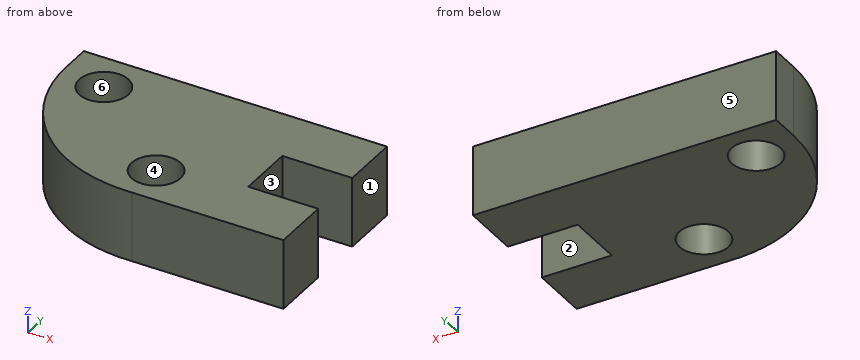
```python
from build123d import *

# Parameters (mm, degrees)
ESQUISSE1_R        = 2.1
BOSS_EXTRU_1_DEPTH = 6


with BuildPart() as part:
    # Esquisse1 → Boss.-Extru.1 (new body)
    with BuildSketch(Plane.XY):
        with BuildLine():
            Line((0, 0), (0, -5.05))
            Line((0, -5.05), (-6, -5.05))
            Line((-6, -5.05), (-6, -10))
            Line((-6, -10), (0, -10))
            Line((0, -10), (0, -15.05))
            Line((0, -15.05), (-13, -15.05))
            ThreePointArc((-13, -15.05), (-22.164162355, -11.534690089), (-26, -2.5))
            Line((-26, -2.5), (-26, 0))
            Line((-26, 0), (0, 0))
        make_face()
        with Locations((-22.2, -3.525)):
            Circle(ESQUISSE1_R, mode=Mode.SUBTRACT)
        with Locations((-13, -11.525)):
            Circle(ESQUISSE1_R, mode=Mode.SUBTRACT)
    extrude(amount=BOSS_EXTRU_1_DEPTH)


solid = part.part
```
Build history of the part. All positions in model axes, mm. Face numbers are marked on the shaded views. A direction names the side the tool comes from. Give positions to 0.01 mm unless a question says otherwise; leave off trailing zeros. Loops run counter-clockwise (first coordinate to the right, second up) from the corner with the lowest first, then second, coordinate; pieces in that order, holes last.
1) Band-saw the part on C-C on z = 2.7. List the corners of the cut face in (x, y) (3 decimals), then the cut area to 3 significant figures.
Values follow:
outline: (-26, -2.5) arc R12.558 ccw to (-13, -15.05) - (0, -15.05) - (0, -10) - (-6, -10) - (-6, -5.05) - (0, -5.05) - (0, 0) - (-26, 0) - close; hole circle Ø4.2 at (-22.2, -3.525); hole circle Ø4.2 at (-13, -11.525)
area: 300 mm2
2) Two-plate mould, pull along X, no slides. Class the marked faces 3, 4, 5 and 6: released by +X, released by -X, zero draft, split by the parting line, or undercut.
Values follow:
face 3: released by +X
face 4: undercut
face 5: zero draft
face 6: undercut
3) Band-saw the part on B-B on y = -12. List the corners of the cut face in (x, z).
Values follow:
outline: (-21.65, 0) - (-15.05, 0) - (-15.05, 6) - (-21.65, 6) - close; (-10.95, 0) - (0, 0) - (0, 6) - (-10.95, 6) - close
4) 3-axis set-ups, long thin cutter, end or side, ignore diameter. For the marked faces 1 and 2: which of +Z, -Z, +X, -X, +Y, -Y reach the whole face in a straight line?
Values follow:
face 1: +Z, -Z, +X, +Y, -Y
face 2: +Z, -Z, +X
5) Probe line 1 along Y through (x, z) = (-13, 4.9) (3 decimals); line 2 along Y through (x, z) = (-2.75, 2.25); line 3 along X through (y, z) = (-3.5, 5.2). List the from-to ranges inside material, lowest first.
Values follow:
line 1: y = -15.05 to -13.625, -9.425 to 0
line 2: y = -15.05 to -10, -5.05 to 0
line 3: x = -25.96 to -24.3, -20.1 to 0
6) Drop flat-ended pins along their axis: P1, Ø3, axis at x = -4, z = 3, coming from the -Y side; P2, Ø4, axis at x = -13, y = -11.525, coming from the -Z side. Give the stop position or say it passes through.
Values follow:
P1: stops at y = -15.05
P2: passes through
7) Band-saw the part on A-A on x = -4. List the corners of the cut face in (y, z), then the cut area to 3 significant figures.
Values follow:
outline: (-15.05, 0) - (-10, 0) - (-10, 6) - (-15.05, 6) - close; (-5.05, 0) - (0, 0) - (0, 6) - (-5.05, 6) - close
area: 60.6 mm2
